Can you work these out from the model? Positions are in its coordinate system, mm. A direction names the side the tool comes from. Give positions to 0.01 mm unless a question says otherwise; leave off trailing zeros. Loops run counter-clockwise (first coordinate to the right, second up) from the corner with the lowest first, then second, coordinate; pieces in that order, holes last. Notation, with made-up numbers: (-13, -1.5) -> (28, -1.5) arc R18 cw to (28, 20.5) -> close; hole circle Ø2 at (38, 20.25). An arc over 180 degrees is marked (long way). Return JSON: item names as keys, results as strings. Group by question number.
Q1. Thinking about a two-plate mould opening in Z: for faces 1 (the flat face through (7, 202, 20)), 2 (the cylindrical face through (7.605, -0.055, -16.313)), 3 (the flat face through (7, 91, -35)), which applies, pulls with the +Z half, pulls with the -Z half, needs draft (parallel to the pull), parting line crosses it, or undercut?
Q2. Will these pins go through, and if not, where does the flat tip stop? pin 1 (8 mm diameter, centred on x = 12.5, z = -10.5, fed in from +Y); pin 2 (4.5 mm diameter, centred on x = 11, y = -21.5, fed in from -Z); pin 3 (8 mm diameter, centred on x = 9.5, z = 22, fed in from +Y).
Q3. Which directions (+Z, -Z, +X, -X, +Y, -Y) give clear straight access to the entire face, cutting with the end or side of a thin tool? Please do faces 4 (the cylindrical face through (8.841, -26.233, 14.804)), 5 (the flat face through (7.605, 9.113, -9.272)), 6 (the flat face through (7, -27, 1)), 7 (the flat face through (7, -31, -15)), 8 (the flat face through (7, -19, 29)).
Q4. Suppose I cut it at B-B, the plane z = -25.5. Please give me the cut outline in (x, y).
Q5. Suppose I cut it at C-C, the plane y = -23. Please give me the cut outline in (x, z), and give its area (3 significant figures).
Q6. Suppose I cut it at D-D, the plane x = 7.5. Count the separate pieces of the cut face and the enclosed holes in it, and give its area (3 significant figures).
Q7. Suppose I cut it at A-A, the plane y = 71. Please give me the cut outline in (x, z).
Q8. I need wall thicknesses on line 1 along X through (y, z) = (-23, -15); line 2 along Z through (x, y) = (1.25, 102); line 3 along Y through (x, z) = (7.5, 13.25). Which ranges of each line are inside material? Lowest first, please. Write a range as [from, to].
Autodesk Inventor part; units mm, degrees
ref_plane "YZ Plane" through (0, 0, 0) normal (1, 0, 0) x (0, 1, 0)
ref_plane "XZ Plane" through (0, 0, 0) normal (0, 1, 0) x (-1, 0, 0)
ref_plane "XY Plane" through (0, 0, 0) normal (0, 0, 1) x (1, 0, 0)
sketch "Esquisse1" plane through (0, 0, 0) normal (1, 0, 0) x (0, 1, 0)
  line L0 (0, 0) -> (122.5, 0)
  line L1 (217, 0) -> (217, 4.1716)
  line L2 (216.4142, 5.5858) -> (187.5858, 34.4142)
  line L3 (186.1716, 35) -> (-6.5, 35)
  line L4 (-9, 32.5) -> (-9, 31.5)
  line L5 (-11.5, 29) -> (-31, 29)
  line L6 (-31, 29) -> (-31, 1)
  line L7 (-31, 1) -> (0, 1)
  line L8 (0, 1) -> (0, 0)
  arc A0 (217, 4.1716) -> (216.4142, 5.5858) centre (215, 4.1716) ccw
  arc A1 (187.5858, 34.4142) -> (186.1716, 35) centre (186.1716, 33) ccw
  arc A2 (-6.5, 35) -> (-9, 32.5) centre (-6.5, 32.5) ccw
  arc A3 (-11.5, 29) -> (-9, 31.5) centre (-11.5, 31.5) ccw
  line L9 (217, 0) -> (217, -4.1716)
  line L10 (216.4142, -5.5858) -> (187.5858, -34.4142)
  line L11 (186.1716, -35) -> (-6.5, -35)
  line L12 (-9, -32.5) -> (-9, -31.5)
  line L13 (-11.5, -29) -> (-31, -29)
  line L14 (-31, -29) -> (-31, -1)
  line L15 (-31, -1) -> (0, -1)
  line L16 (0, -1) -> (0, 0)
  arc A4 (216.4142, -5.5858) -> (217, -4.1716) centre (215, -4.1716) ccw
  arc A5 (186.1716, -35) -> (187.5858, -34.4142) centre (186.1716, -33) ccw
  arc A6 (-9, -32.5) -> (-6.5, -35) centre (-6.5, -32.5) ccw
  arc A7 (-9, -31.5) -> (-11.5, -29) centre (-11.5, -31.5) ccw
  point P0 (217, 5)
  point P1 (217, -5)
  dimension "d0" = 70
  dimension "d1" = 10
  dimension "d2" = 45
  dimension "d3" = 31
  dimension "d4" = 22
  dimension "d5" = 217
  dimension "d6" = 58
  dimension "d7" = 2
  dimension "d8" = 2
  dimension "d9" = 2.5
extrude "Extrusion1" add sketch "Esquisse1" along normal blind 15
sketch "Esquisse2" plane through (15, 0, 0) normal (1, 0, 0) x (0, 0, -1)
  line L0 (0, 210) -> (0, 210)
  line L1 (15, 49) -> (-15, 49)
  line L2 (4.1716, 217) -> (-4.1716, 217)
  arc A0 (0, 210) -> (-15, 195) centre (0, 195) ccw
  arc A1 (15, 195) -> (0, 210) centre (0, 195) ccw
  line L3 (1, -31) -> (29, -31)
  line L4 (-3.5355, 14.8492) -> (-14.8492, 3.5355)
  line L5 (-14.8492, -3.5355) -> (-3.5355, -14.8492)
  line L6 (3.5355, -14.8492) -> (14.8492, -3.5355)
  line L7 (14.8492, 3.5355) -> (3.5355, 14.8492)
  arc A2 (3.5355, 14.8492) -> (-3.5355, 14.8492) centre (0, 11.3137) ccw
  arc A3 (14.8492, -3.5355) -> (14.8492, 3.5355) centre (11.3137, 0) ccw
  arc A4 (-3.5355, -14.8492) -> (3.5355, -14.8492) centre (0, -11.3137) ccw
  arc A5 (-14.8492, 3.5355) -> (-14.8492, -3.5355) centre (-11.3137, 0) ccw
  line L8 (-35, 186.1716) -> (-35, -6.5)
  line L9 (-1, 0) -> (1, 0)
  arc A6 (15, 49) -> (15, 59) centre (15, 54) ccw
  arc A7 (-15, 59) -> (-15, 49) centre (-15, 54) ccw
  arc A8 (-15, 76) -> (-15, 66) centre (-15, 71) ccw
  line L10 (-15, 59) -> (-15, 66)
  line L11 (-15, 76) -> (-15, 195)
  arc A9 (15, 66) -> (15, 76) centre (15, 71) ccw
  line L12 (15, 195) -> (15, 76)
  line L13 (15, 66) -> (15, 59)
  point P0 (0, 0)
  point P1 (-15, 210)
  point P2 (15, 210)
  point P3 (0, 18.3848)
  point P4 (-18.3848, 0)
  point P5 (18.3848, 0)
  point P6 (0, 0)
  point P7 (0, 0)
  dimension "d12" = 30
  dimension "d14" = 7
  dimension "d15" = 15
  dimension "d16" = 80
  dimension "d17" = 26
  dimension "d18" = 26
  dimension "d19" = 5
  dimension "d20" = 45
  dimension "d21" = 10
  dimension "d22" = 10
  dimension "d23" = 10
  dimension "d24" = 12
  dimension "d25" = 10
  dimension "d26" = 30
  dimension "d27" = 15
extrude "Extrusion2" cut sketch "Esquisse2" against normal through all
sketch "Esquisse3" plane through (0, -31, 29) normal (0, 0, 1) x (1, 0, 0)
  line L0 (0, 0) -> (0, 19.5)
  line L1 (0, 0) -> (15, 0)
  point P0 (0, 31)
  point P1 (7.5, 8)
  dimension "d30" = 7.5
  dimension "d31" = 8
hole "Perçage1" at (7.5, -23, 29) direction (0, 0, -1) diameter 7 end through all
properties part number "came"
Ans:
{
 "1": {"face 1": "pulls with the +Z half", "face 2": "undercut", "face 3": "pulls with the -Z half"},
 "2": {"pin 1": "stops at y = 215.5", "pin 2": "stops at z = -29", "pin 3": "stops at y = 204"},
 "3": {"face 4": "+Z, -Z", "face 5": "+X, -X", "face 6": "+X, -X, -Y", "face 7": "+Z, -Z, +X, -X, -Y", "face 8": "+Z, +X, -X, -Y"},
 "4": {"outline": "(0, -31) -> (15, -31) -> (15, 196.5) -> (0, 196.5) -> close; hole circle Ø7 at (7.5, -23)"},
 "5": {"outline": "(0, -29) -> (4, -29) -> (4, -1) -> (0, -1) -> close; (0, 1) -> (4, 1) -> (4, 29) -> (0, 29) -> close; (11, -29) -> (15, -29) -> (15, -1) -> (11, -1) -> close; (11, 1) -> (15, 1) -> (15, 29) -> (11, 29) -> close", "area": "448 mm^2"},
 "6": {"separate pieces": "3", "enclosed holes": "1", "area": "10,200 mm^2"},
 "7": {"outline": "(0, -35) -> (15, -35) -> (15, -20) -> (0, -20) -> close; (0, 20) -> (15, 20) -> (15, 35) -> (0, 35) -> close"},
 "8": {"line 1": "x = [0, 4], [11, 15]", "line 2": "z = [-35, -15], [15, 35]", "line 3": "y = [-31, -26.5], [-19.5, -5.13], [5.13, 49], [202.03, 208.75]"}
}
